from build123d import *

# Parameters (mm, degrees)
SKETCH1_R           = 2.838382548
BOSS_EXTRUDE2_DEPTH = 12.7


with BuildPart() as part:
    # Sketch1 → Boss-Extrude2 (new body)
    with BuildSketch(Plane.XY):
        with BuildLine():
            Line((-26.824587008, 88.76822773), (25.274610138, 81.274279665))
            Line((25.274610138, 81.274279665), (66.134216336, 66.398380962))
            ThreePointArc((66.134216336, 66.398380962), (74.236045161, 59.4504343), (80.201058977, 50.599886109))
            Line((80.201058977, 50.599886109), (59.165982949, -5.321540814))
            ThreePointArc((59.165982949, -5.321540814), (52.522719394, -12.417211597), (42.807825757, -12.737111817))
            Line((42.807825757, -12.737111817), (31.132290646, -8.345310995))
            ThreePointArc((31.132290646, -8.345310995), (29.649176446, -5.073679556), (32.920807884, -3.590565356))
            ThreePointArc((32.920807884, -3.590565356), (34.228479037, -3.692067968), (35.539646393, -3.725932272))
            ThreePointArc((35.539646393, -3.725932272), (59.225238989, 12.500589471), (52.648250228, 40.447870615))
            ThreePointArc((52.648250228, 40.447870615), (44.71312465, 45.359660325), (35.539646393, 47.074067728))
            Line((35.539646393, 47.074067728), (9.696061009, 47.807757753))
            ThreePointArc((9.696061009, 47.807757753), (-3.214919538, 50.169926542), (-14.819759488, 56.301887878))
            Line((-14.819759488, 56.301887878), (-37.452223969, 73.106391791))
            Line((-37.452223969, 73.106391791), (-26.824587008, 88.76822773))
        make_face()
        with Locations((20.390142766, 51.502972215)):
            Circle(SKETCH1_R, mode=Mode.SUBTRACT)
        with BuildLine():
            Line((24.516957739, 66.398380962), (-13.583042261, 71.878684632))
            ThreePointArc((-13.583042261, 71.878684632), (-16.273658443, 75.473379968), (-12.678963107, 78.16399615))
            Line((-12.678963107, 78.16399615), (25.421036893, 72.68369248))
            ThreePointArc((25.421036893, 72.68369248), (28.111653075, 69.088997144), (24.516957739, 66.398380962))
        make_face(mode=Mode.SUBTRACT)
    extrude(amount=BOSS_EXTRUDE2_DEPTH)


solid = part.part
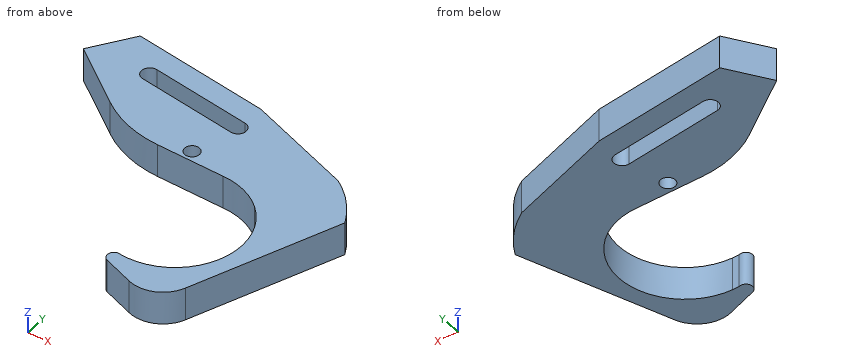
Geometry check sheet. Reference: the model listing, model coordinates, mm. Round coordinates to 2 decimals unless told otherwise and drop trailing zeros. Order: outer loops, then holes, each group sorted by start corner. A loop starts at its lowest first (then second) coordinate and runs counter-clockwise, first axis right, second up. Notation, with made-up numbers: M -9,-14.5 L 50,-14.5 A29 ccw 50,24.5 Z; hole C 61.25,71.25 d5. An arc over 180 degrees is marked long. Answer in a Markdown table with one row per item.
(1) Sectioned sample at B-B, the plane y = 70. Record the cut outline in (x, z), and give its area (3 significant figures).
Responses:
| item | result |
|---|---|
| outline | M -33.27,0 L -0.52,0 L -0.52,12.7 L -33.27,12.7 Z; M 28.11,0 L 56.24,0 L 56.24,12.7 L 28.11,12.7 Z |
| area | 773 mm² |
(2) Sectioned sample at A-A, the plane x = -11. Record the cut outline in (y, z).
Responses:
| item | result |
|---|---|
| outline | M 53.77,0 L 71.51,0 L 71.51,12.7 L 53.77,12.7 Z; M 77.92,0 L 86.49,0 L 86.49,12.7 L 77.92,12.7 Z |
(3) Sectioned sample at D-D, the plane z = 9.5. Record the cut outline in (x, y) (3 decimals), and give its area (3 significant figures).
Responses:
| item | result |
|---|---|
| outline | M -37.452,73.106 L -14.82,56.302 A43.18 ccw 9.696,47.808 L 35.54,47.074 A25.4 cw long 32.921,-3.591 A2.54 ccw 31.132,-8.345 L 42.808,-12.737 A12.7 ccw 59.166,-5.322 L 80.201,50.6 A39.815 ccw 66.134,66.398 L 25.275,81.274 L -26.825,88.768 Z; hole M -13.583,71.879 L 24.517,66.398 A3.175 ccw 25.421,72.684 L -12.679,78.164 A3.175 ccw Z; hole C 20.39,51.503 d5.677 |
| area | 3,730 mm² |
(4) Go/stop test with flat-tipped pins: P1, Ø1, axis at y = 63, z = 9, coming from the -X side; P2, Ø2, axis at x = -15.5, z = 2, coming from the -Y side; P3, Ø4, axis at x = 28, z = 2, coming from the +Y side; P4, Ø8, axis at x = 57, y = 31.5, coming from the +Z side. Record where each tip stops, or that it passes through.
Responses:
| item | result |
|---|---|
| P1 | stops at x = -24.51 |
| P2 | stops at y = 56.07 |
| P3 | stops at y = 81.01 |
| P4 | stops at z = 12.7 |
(5) Scan lines: probe 1 along Y at (x, z) = (-11.5, 5.5); probe 2 along Y at (x, z) = (2, 1.75); probe 3 along X at (y, z) = (23, 0.75). Record each from-to range of solid material in increasing order. Write a range as from..to.
Responses:
| item | result |
|---|---|
| probe 1 | y = 54.07..71.58, 77.99..86.56 |
| probe 2 | y = 48.72..69.64, 76.05..84.62 |
| probe 3 | x = 60.91..69.82 |
(6) Sectioned sample at C-C, the plane x = 20.5. Record the cut outline in (y, z).
Responses:
| item | result |
|---|---|
| outline | M 47.5,0 L 48.67,0 L 48.67,12.7 L 47.5,12.7 Z; M 54.34,0 L 66.98,0 L 66.98,12.7 L 54.34,12.7 Z; M 73.39,0 L 81.96,0 L 81.96,12.7 L 73.39,12.7 Z |
